CAD build for the part. Positions are in the model's coordinates, mm. Coordinates: 2 decimals unless noted, no trailing zeros. Order: outer loops, then holes, each group sorted by start corner. A loop starts at its lowest first (then second) coordinate and runs counter-clockwise, first axis right, second up. Notation, with made-up numbers: (-19.5, 78) - (-10.5, 78) arc R18 cw to (-10.5, 83) - close; hole circle Ø9 at (-20, 9.25). An arc over 180 degrees is marked (long way). Write each question's results on one line, items separated by ' | '. Start each with the question number.
Q1. Wall check: probe 1 along X at (y, z) = (214, 0); probe 2 along Z at (x, y) = (4.5, 19). Give the ranges that are in metal, low to high.
Q2. Pin check, flat tips, straight feed: P1, Ø8, axis at x = 5, y = 32.5, coming from the +Z side; P2, Ø1, axis at x = 6, y = 234.5, coming from the -Z side; P3, Ø2, axis at y = 78.5, z = -42, coming from the -X side. Stop position of each tip, or through.
Q3. Band-saw the part on A-A, the plane y = 130. Write the cut outline in (x, z) (3 decimals), then the cut area to 3 significant figures.
Q4. Band-saw the part on D-D, the plane y = 58. Write the cut outline in (x, z).
Q5. Band-saw the part on B-B, the plane x = 0. Write the cut outline in (y, z), then the cut area to 3 significant figures.
Q6. Band-saw the part on C-C, the plane z = -56.5. Write the cut outline in (x, y).
```python
from build123d import *

# Parameters (mm, degrees)
SKIZZE2_R                       = 10
AUFSATZ_LINEAR_AUSTRAGEN1_DEPTH = 295
SKIZZE7_W                       = 10.134043554
SKIZZE7_H                       = 150
AUFSATZ_LINEAR_AUSTRAGEN2_DEPTH = 70
AUFSATZ_LINEAR_AUSTRAGEN2_DRAFT = -1


with BuildPart() as part:
    # Skizze2 → Aufsatz-Linear austragen1 (new body)
    with BuildSketch(Plane(origin=(0, 0, 0), x_dir=(1, 0, 0), z_dir=(0, 1, 0))):
        with Locations(Location((0, 0, 0), (0, 0, 270))):
            Circle(SKIZZE2_R)
    extrude(amount=AUFSATZ_LINEAR_AUSTRAGEN1_DEPTH)


with BuildPart() as aufsatz_linear_austragen2_tool:
    # Skizze7 → Aufsatz-Linear austragen2 (with draft: the straight prism first)
    with BuildSketch(Plane.XY):
        with Locations((0, 147.5)):
            Rectangle(SKIZZE7_W, SKIZZE7_H)
    extrude(amount=-AUFSATZ_LINEAR_AUSTRAGEN2_DEPTH)
    # Aufsatz-Linear austragen2: the draft: its side faces are tilted about the plane it starts from
    aufsatz_linear_austragen2_sides = [aufsatz_linear_austragen2_tool.faces().sort_by_distance(p)[0] for p in [
        (0, 222.5, -35),
        (-5.067021777, 147.5, -35),
        (0, 72.5, -35),
        (5.067021777, 147.5, -35),
    ]]
    draft(aufsatz_linear_austragen2_sides, Plane.XY, AUFSATZ_LINEAR_AUSTRAGEN2_DRAFT)


with BuildPart() as part_1:
    add(part.part)

    # Aufsatz-Linear austragen2: add aufsatz_linear_austragen2_tool
    add(aufsatz_linear_austragen2_tool.part)


solid = part_1.part
```
Results below:
1) probe 1: x = -10 to 10 | probe 2: z = -8.93 to 8.93
2) P1: stops at z = 9.95 | P2: stops at z = -8.35 | P3: stops at x = -4.35
3) outline: (-4.915, -8.709) - (-3.845, -70) - (3.845, -70) - (4.915, -8.709) arc R10 ccw (long way) to start | area: 843 mm²
4) outline: circle Ø20 at (0, 0)
5) outline: (0, -10) - (72.67, -10) - (73.72, -70) - (221.28, -70) - (222.33, -10) - (295, -10) - (295, 10) - (0, 10) - close | area: 14,800 mm²
6) outline: (-4.08, 73.49) - (4.08, 73.49) - (4.08, 221.51) - (-4.08, 221.51) - close
